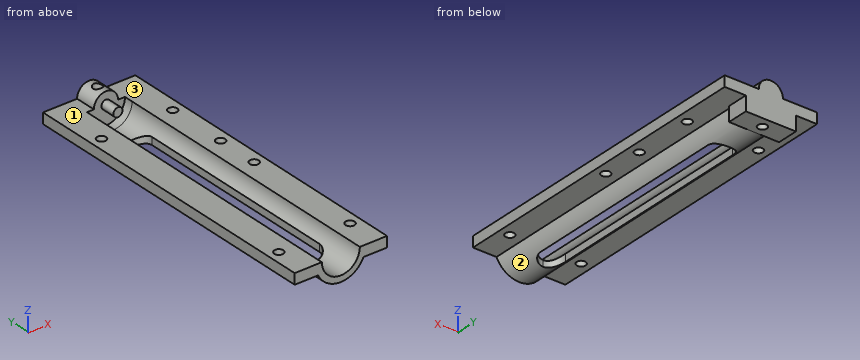
```python
from build123d import *

# Parameters (mm, degrees)
SKETCH1_R                = 8.3
SKETCH1_R_2              = 6.3
BOSS_EXTRUDE1_DEPTH      = 95
SKETCH3_R                = 8.3
BOSS_EXTRUDE2_DEPTH      = 3
SKETCH5_W                = 16.6
SKETCH5_H                = 16.6
BOSS_EXTRUDE4_DEPTH      = 7
CUT_EXTRUDE1_DEPTH       = 107.627623063
FILLET1_R                = 4.1
SKETCH4_R                = 6.3
SKETCH4_R_2              = 1.5
CUT_EXTRUDE3_DEPTH       = 3
BOSS_EXTRUDE6_START      = 2
SKETCH8_R                = 1.5
BOSS_EXTRUDE6_DEPTH      = 2
BOSS_EXTRUDE7_START      = -0.774045
BOSS_EXTRUDE7_DEPTH      = 7.774045
F_3_0_3_DIAMETER_HOLE1_D = 3
F_3_0_3_DIAMETER_HOLE2_D = 3
F_3_0_3_DIAMETER_HOLE3_D = 3
CUT_EXTRUDE4_DEPTH       = 107.432983617


with BuildPart() as part:
    # Sketch1 → Boss-Extrude1 (new body)
    with BuildSketch(Plane(origin=(0, 0, 0), x_dir=(1, 0, 0), z_dir=(0, 1, 0))):
        with Locations(Location((0, 0, 0), (0, 0, 270))):
            Circle(SKETCH1_R)
        with Locations(Location((0, 0, 0), (0, 0, 270))):
            Circle(SKETCH1_R_2, mode=Mode.SUBTRACT)
    extrude(amount=BOSS_EXTRUDE1_DEPTH)

    # Sketch3 → Boss-Extrude2 (add)
    with BuildSketch(Plane(origin=(0, 95, 0), x_dir=(1, 0, 0), z_dir=(0, 1, 0))):
        with Locations(Location((0, 0, 0), (0, 0, 270))):
            Circle(SKETCH3_R)
    extrude(amount=BOSS_EXTRUDE2_DEPTH)

    # Sketch5 → Boss-Extrude4 (add)
    with BuildSketch(Plane(origin=(0, 98, 0), x_dir=(1, 0, 0), z_dir=(0, 1, 0))):
        Rectangle(SKETCH5_W, SKETCH5_H)
    extrude(amount=BOSS_EXTRUDE4_DEPTH)

    # Sketch6 → Cut-Extrude1 (cut, through all)
    with BuildSketch(Plane.XY.offset(8.3)):
        Polygon((4.1, 10), (0, 10), (-4.1, 10), (-4.1, 88), (4.1, 88), align=None)
    extrude(amount=-CUT_EXTRUDE1_DEPTH, mode=Mode.SUBTRACT)

    # Fillet1
    fillet1_edges = [part.edges().sort_by_distance(p)[0] for p in [
        (4.1, 88, 5.999975859),
        (4.1, 88, -5.999975859),
        (-4.1, 88, 5.999975859),
        (-4.1, 88, -5.999975859),
        (4.1, 10, -5.999975859),
        (4.1, 10, 5.999975859),
        (-4.1, 10, -5.999975859),
        (-4.1, 10, 5.999975859),
    ]]
    fillet(fillet1_edges, radius=FILLET1_R - 0.0001)  # a hair under: the kernel refuses the full size

    # Sketch4 → Cut-Extrude3 (cut)
    with BuildSketch(Plane(origin=(0, 95, 0), x_dir=(-1, 0, 0), z_dir=(0, -1, 0))):
        with Locations(Location((0, 0, 0), (0, 0, 90))):
            Circle(SKETCH4_R)
        with Locations(Location((0, 0, 0), (0, 0, 90))):
            Circle(SKETCH4_R_2, mode=Mode.SUBTRACT)
    extrude(amount=-CUT_EXTRUDE3_DEPTH, mode=Mode.SUBTRACT)

    # Sketch8 → Boss-Extrude6 (add)
    with BuildSketch(Plane(origin=(0, 95, 0), x_dir=(-1, 0, 0), z_dir=(0, -1, 0)).offset(BOSS_EXTRUDE6_START)):
        with Locations(Location((0, 0, 0), (0, 0, 90))):
            Circle(SKETCH8_R)
    extrude(amount=-BOSS_EXTRUDE6_DEPTH)

    # Sketch9 → Boss-Extrude7 (add)
    with BuildSketch(Plane.ZY.offset(8.3).offset(BOSS_EXTRUDE7_START)):
        Polygon((0, 0), (3.5, 0), (3.5, 105), (-3.5, 105), (-3.5, 0), align=None)
    boss_extrude7 = extrude(amount=BOSS_EXTRUDE7_DEPTH)

    # Mirror1: Boss-Extrude7 across plane
    add(boss_extrude7.mirror(Plane(origin=(0, 0, 0), x_dir=(0, 0, 1), z_dir=(1, 0, 0))))

    # Ø3.0 (3) Diameter Hole1 (through all)
    with Locations(Plane.XY.offset(8.3)):
        with Locations((0, 101.5)):
            Hole(F_3_0_3_DIAMETER_HOLE1_D / 2)

    # Ø3.0 (3) Diameter Hole2 (through all)
    with Locations(Plane.XY.offset(3.5)):
        with Locations((11.8, 85), (11.8, 11)):
            f_3_0_3_diameter_hole2 = Hole(F_3_0_3_DIAMETER_HOLE2_D / 2)

    # Ø3.0 (3) Diameter Hole3 (through all)
    with Locations(Plane(origin=(0, 0, -3.5), x_dir=(-1, 0, 0), z_dir=(0, 0, -1))):
        with Locations((-11.8, 65), (-11.8, 51)):
            Hole(F_3_0_3_DIAMETER_HOLE3_D / 2)

    # Mirror2: Ø3.0 (3) Diameter Hole2 across plane
    add(f_3_0_3_diameter_hole2.mirror(Plane(origin=(0, 0, 0), x_dir=(0, 0, 1), z_dir=(1, 0, 0))), mode=Mode.SUBTRACT)

    # Sketch17 → Cut-Extrude4 (cut, through all)
    with BuildSketch(Plane(origin=(0, 0, 0), x_dir=(-1, 0, 0), z_dir=(0, -1, 0))):
        with BuildLine():
            Line((15.3, -73.411355502), (15.3, 0))
            Line((15.3, 0), (15.3, 8.3))
            Line((15.3, 8.3), (-15.3, 8.3))
            Line((-15.3, 8.3), (-15.3, -8.3))
            Line((-15.3, -8.3), (15.3, -8.3))
            Line((15.3, -8.3), (15.3, 0))
            Line((15.3, 0), (4, 0))
            ThreePointArc((4, 0), (0, -4), (-4, 0))
            Line((-4, 0), (-15.3, 0))
            Line((-15.3, 0), (-88.711355502, 0))
            Line((-88.711355502, 0), (-173.375060896, -119.954013921))
            Line((-173.375060896, -119.954013921), (-69.363705394, -193.365369423))
            Line((-69.363705394, -193.365369423), (15.3, -73.411355502))
        make_face()
    extrude(amount=-CUT_EXTRUDE4_DEPTH, mode=Mode.SUBTRACT)


with BuildPart() as cut_extrude4_kept_piece:
    # of the separate pieces the step leaves, the one the design keeps (cut_extrude4_pieces_kept)
    add(part.part.solids().sort_by_distance((15.3, 0, -3.5))[0])


solid = cut_extrude4_kept_piece.part
```
Input: part model. Units: mm. Frame: model coordinates. Face numbers are marked on the shaded views. A direction names the side the tool comes from. Give positions to 0.01 mm unless a question says otherwise; leave off trailing zeros. Loops run counter-clockwise (first coordinate to the right, second up) from the corner with the lowest first, then second, coordinate; pieces in that order, holes last.
1) Section query D-D on y = 11. Return the cut outline in (x, z), and give its area (3 significant figures).
A:
outline: (-15.3, -3.5) - (-13.3, -3.5) - (-13.3, 0) - (-15.3, 0) - close; (-10.3, -3.5) - (-7.53, -3.5) arc R8.3 ccw to (-2.68, -7.85) - (-2.68, -5.7) arc R6.3 cw to (-6.3, 0) - (-10.3, 0) - close; (2.68, -7.85) arc R8.3 ccw to (7.53, -3.5) - (10.3, -3.5) - (10.3, 0) - (6.3, 0) arc R6.3 cw to (2.68, -5.7) - close; (13.3, -3.5) - (15.3, -3.5) - (15.3, 0) - (13.3, 0) - close
area: 64.6 mm2
2) Section query B-B on x = 11.8. Return the cut outline in (y, z).
A:
outline: (0, -3.5) - (9.5, -3.5) - (9.5, 0) - (0, 0) - close; (12.5, -3.5) - (49.5, -3.5) - (49.5, 0) - (12.5, 0) - close; (52.5, -3.5) - (63.5, -3.5) - (63.5, 0) - (52.5, 0) - close; (66.5, -3.5) - (83.5, -3.5) - (83.5, 0) - (66.5, 0) - close; (86.5, -3.5) - (105, -3.5) - (105, 0) - (86.5, 0) - close
3) Line query: L1, parallel to Y at x = 11.8, z = -2.8; L2, parallel to X at y = 10, z = -0.5; L3, parallel to X at y = 65, z = -1.5. Output: solid intervals per line, ascending.
A:
L1: y = 0 to 9.5, 12.5 to 49.5, 52.5 to 63.5, 66.5 to 83.5, 86.5 to 105
L2: x = -15.3 to -12.92, -10.68 to -6.28, 6.28 to 10.68, 12.92 to 15.3
L3: x = -15.3 to -6.12, 6.12 to 10.3, 13.3 to 15.3
4) Section query A-A on y = 27.5. Return the cut outline in (x, z), and give its area (3 significant figures).
A:
outline: (-15.3, -3.5) - (-7.53, -3.5) arc R8.3 ccw to (-4.1, -7.22) - (-4.1, -4.78) arc R6.3 cw to (-6.3, 0) - (-15.3, 0) - close; (4.1, -7.22) arc R8.3 ccw to (7.53, -3.5) - (15.3, -3.5) - (15.3, 0) - (6.3, 0) arc R6.3 cw to (4.1, -4.78) - close
area: 79.2 mm2
5) Section query C-C on y = 65. Return the cut outline in (x, z).
A:
outline: (-15.3, -3.5) - (-7.53, -3.5) arc R8.3 ccw to (-4.1, -7.22) - (-4.1, -4.78) arc R6.3 cw to (-6.3, 0) - (-15.3, 0) - close; (4.1, -7.22) arc R8.3 ccw to (7.53, -3.5) - (10.3, -3.5) - (10.3, 0) - (6.3, 0) arc R6.3 cw to (4.1, -4.78) - close; (13.3, -3.5) - (15.3, -3.5) - (15.3, 0) - (13.3, 0) - close
6) Reachability of the marked faces 1, 2 and 3 from +Z, -Z, +X, -X, +Y, -Y: full face, straight path, thin tool, end or side. Return the list, or none.
A:
face 1: +Z, -X, +Y, -Y
face 2: -Z, -Y
face 3: +Z, +X, +Y, -Y
7) Contact query for flat-ended pins moving along their axis: pin 1 (4 mm diameter, centred on x = 11.8, y = 11, fed in from -Z); pin 2 (3.5 mm diameter, centred on x = -11.8, y = 85, fed in from +Z); pin 3 (6 mm diameter, centred on x = -8, z = -5, fed in from -Y); pin 4 (2.5 mm diameter, centred on y = 38.5, z = -6, fed in from -X). Output: stop coordinate, or through.
A:
pin 1: stops at z = -3.5
pin 2: stops at z = 0
pin 3: stops at y = 0
pin 4: stops at x = -6.81
